from build123d import *

# Parameters (mm, degrees)
F0_W     = 5.8
F0_H     = 2
F0_H_2   = 2.8
F1_DEPTH = 3
F2_DEPTH = 60
F3_SIZE  = 1.99999


# Not quite as in the source:
# - a fillet or chamfer is up to 0.001 mm smaller than in the source, because OpenCascade refuses the exact size
# - a feature names something its author has since deleted; it is built from what else it names


with BuildPart() as f1:
    # F0 (on Top) → F1 (new body)
    with BuildSketch(Plane.XY):
        with Locations((-14.8613960065, 7.2783571027)):
            Rectangle(F0_W, F0_H)
        with Locations((-14.8613960065, 4.8783571027)):
            Rectangle(F0_W, F0_H_2)
    extrude(amount=F1_DEPTH)

    # F0 (on Top) → F2 (join)
    with BuildSketch(Plane.XY):
        with Locations((-14.8613960065, 4.8783571027)):
            Rectangle(F0_W, F0_H_2)
    extrude(amount=F2_DEPTH)

    # F3 (size 2 in the source; OpenCascade refuses exactly that, so slightly less here)
    f3_edges = [f1.edges().sort_by_distance(p)[0] for p in [
        (-14.861396, 8.278357, 3),
    ]]
    chamfer(f3_edges, length=F3_SIZE)


solid = f1.part
Geometry: final body of the model. Coordinates: model frame, mm. A direction names the side the tool comes from. Coordinates: 2 decimals unless noted, no trailing zeros. Order: outer loops, then holes, each group sorted by start corner. A loop starts at its lowest first (then second) coordinate and runs counter-clockwise, first axis right, second up.
(1) Section query B-B (z = 48). Return the cut outline in (x, y), plus the area to 3 significant figures.
(2) Section query C-C (y = 7.4). Return the cut outline in (x, z).
(3) Material intervals for probe 1 along Y at (x, z) = (-16.2, 47.5); probe 2 along Z at (x, y) = (-17.35, 6.6); probe 3 along Z at (x, y) = (-13.9, 7.1), sorted ascending.
(4) Access query for faces 1 (the face through (-15, 6.278, 31)), 2 (the face through (-15, 6, 0)). Directions: +Z, -Z, +X, -X, +Y, -Y. A direction counts if a zero-diameter tool reaches every point of the face in a straight line with its end or side. Return the directions, or none.
(5) First-contact query: pin 1 (2 mm diameter, centred on y = 6.5, z = 12, fed in from +X). Flat tip, straight axial feed; report the tip coordinate or a pass-through.
Solution:
1. outline: (-17.76, 3.48) - (-11.96, 3.48) - (-11.96, 6.28) - (-17.76, 6.28) - close
1. area: 16.2 mm2
2. outline: (-17.76, 0) - (-11.96, 0) - (-11.96, 1.88) - (-17.76, 1.88) - close
3. probe 1: y = 3.48 to 6.28
3. probe 2: z = 0 to 2.68
3. probe 3: z = 0 to 2.18
4. face 1: +Z, +X, -X, +Y
4. face 2: -Z, +X, -X, +Y, -Y
5. pin 1: stops at x = -11.96
